Check sheet for the drawn part. Datum: minimum x, y, z corner. Units: mm. A direction names the side the tool comes from. Give positions to 0.01 mm unless a question says otherwise; leave off trailing zeros. Order: outer loops, then holes, each group sorted by start corner. A loop starts at its lowest first (then second) coordinate and runs counter-clockwise, first axis right, second up. Notation, with made-up numbers: (35.25, 41) -> (58.25, 41) arc R25 cw to (58.25, 68) -> close; hole circle Ø1 at (55.5, 31.5). An arc over 180 degrees is marked (long way). Answer in a Markdown table with one row per item. Add a question column.
(1) Cross-section at D-D (z = 23.5). Record the cut outline in (x, y), then the cut area to 3 significant figures.
(2) Go/stop test with flat-tipped pins: pin 1 (1 mm diameter, centred on y = 11.5, z = 67.5, fed in from -X); pin 2 (12 mm diameter, centred on x = 47, z = 31.5, fed in from -Y). Record where each tip stops, or that it passes through.
(3) Cross-section at A-A (z = 38.1). Record the cut outline in (x, y), then the cut area to 3 significant figures.
(4) Thickness scan on L1, parallel to Y at x = 33, z = 38.1; L2, parallel to Y at x = 69, z = 38.1; L3, parallel to Z at x = 48, y = 38. Record the ranges inside material, lowest first. Write a range as [from, to].
(5) Cross-section at C-C (x = 20). Record the cut outline in (y, z).
(6) Set-up check for the marked faces 1 and 2: record each of +Z, -Z, +X, -X, +Y, -Y from which the full face is reachable in a straight line by a thin tool's end or side.
(7) Release check for a two-part mould opening along Y. For the marked faces 3, 4 and 5 record: released by +Y, released by -Y, zero draft, split by the parting line, or undercut.
(8) Cross-section at B-B (y = 38.1). Record the cut outline in (x, z).
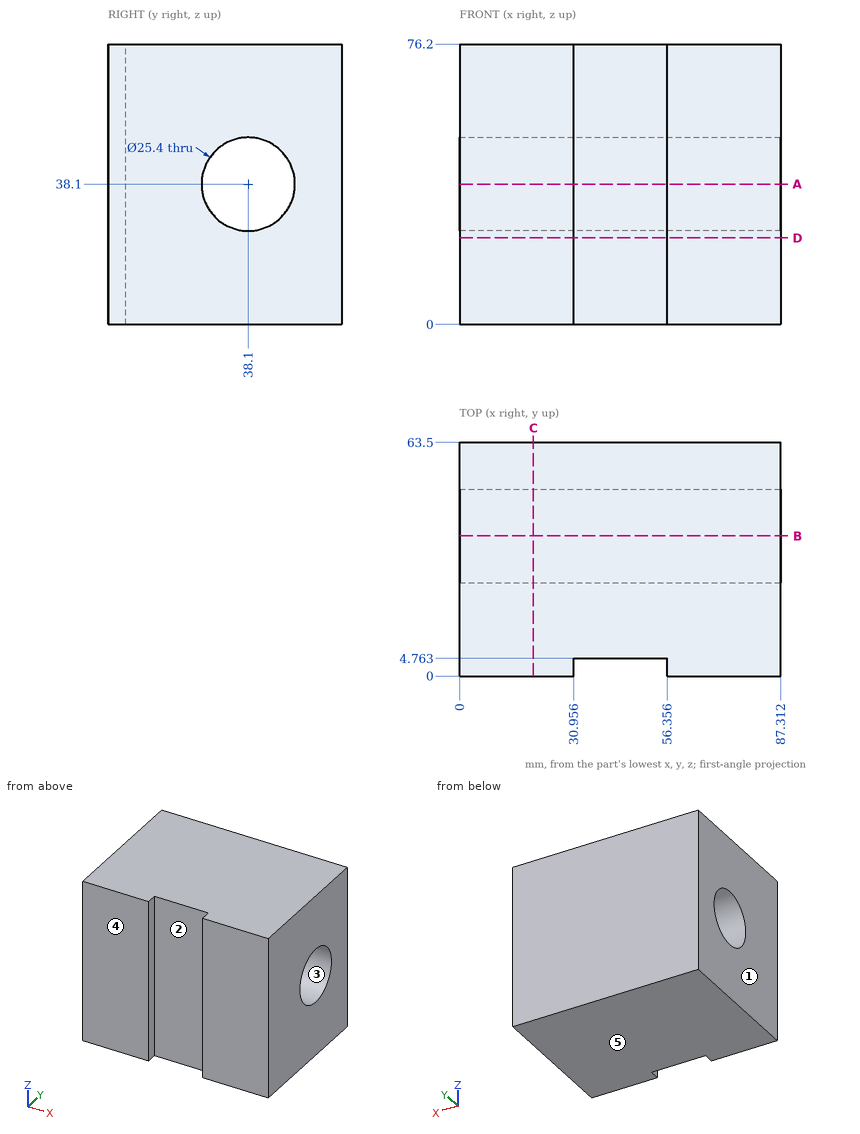
Answer below:
| question | item | result |
|---|---|---|
| 1 | outline | (0, 0) -> (30.96, 0) -> (30.96, 4.76) -> (56.36, 4.76) -> (56.36, 0) -> (87.31, 0) -> (87.31, 63.5) -> (0, 63.5) -> close |
| 1 | area | 5,420 mm² |
| 2 | pin 1 | stops at x = 0 |
| 2 | pin 2 | stops at y = 4.76 |
| 3 | outline | (0, 0) -> (30.96, 0) -> (30.96, 4.76) -> (56.36, 4.76) -> (56.36, 0) -> (87.31, 0) -> (87.31, 25.4) -> (0, 25.4) -> close; (0, 50.8) -> (87.31, 50.8) -> (87.31, 63.5) -> (0, 63.5) -> close |
| 3 | area | 3,210 mm² |
| 4 | L1 | y = [4.76, 25.4], [50.8, 63.5] |
| 4 | L2 | y = [0, 25.4], [50.8, 63.5] |
| 4 | L3 | z = [0, 25.4], [50.8, 76.2] |
| 5 | outline | (0, 0) -> (63.5, 0) -> (63.5, 76.2) -> (0, 76.2) -> close; hole circle Ø25.4 at (38.1, 38.1) |
| 6 | face 1 | +Z, -Z, -X, +Y, -Y |
| 6 | face 2 | +Z, -Z, -Y |
| 7 | face 3 | undercut |
| 7 | face 4 | released by -Y |
| 7 | face 5 | zero draft |
| 8 | outline | (0, 0) -> (87.31, 0) -> (87.31, 25.4) -> (0, 25.4) -> close; (0, 50.8) -> (87.31, 50.8) -> (87.31, 76.2) -> (0, 76.2) -> close |
